```python
from build123d import *

# Parameters (mm, degrees)
SKETCH2_R           = 3.175
BOSS_EXTRUDE2_DEPTH = 25.4
SKETCH3_R           = 4.7625
CUT_EXTRUDE1_DEPTH  = 14.2875


with BuildPart() as part:
    # Sketch2 → Boss-Extrude2 (new body)
    with BuildSketch(Plane(origin=(0, 0, 0), x_dir=(1, 0, 0), z_dir=(0, 1, 0))):
        with BuildLine():
            Line((-15.875, 12.7), (-15.875, -12.7))
            Line((-15.875, -12.7), (15.875, -12.7))
            ThreePointArc((15.875, -12.7), (3.175, 0), (15.875, 12.7))
            Line((15.875, 12.7), (-15.875, 12.7))
        make_face()
        with Locations((-6.35, 0)):
            Circle(SKETCH2_R, mode=Mode.SUBTRACT)
    extrude(amount=BOSS_EXTRUDE2_DEPTH)

    # Sketch3 → Cut-Extrude1 (cut)
    with BuildSketch(Plane.ZY.offset(15.875)):
        with Locations((0, 12.7)):
            Circle(SKETCH3_R)
    extrude(amount=-CUT_EXTRUDE1_DEPTH, mode=Mode.SUBTRACT)


solid = part.part
```
Geometry check sheet. Reference: the model listing, model coordinates, mm. A direction names the side the tool comes from. Round coordinates to 2 decimals unless told otherwise and drop trailing zeros. Loops run counter-clockwise (first coordinate to the right, second up) from the corner with the lowest first, then second, coordinate; pieces in that order, holes last. Notation, with made-up numbers: M 82,46.25 L 104,46.25 A4 ccw 104,51.25 Z; hole C -25.75,49 d8. An arc over 180 degrees is marked long. Return JSON: item names as keys, results as strings. Group by question number.
(1) Mould release check, pull along Z, two halves, no side actions. Record for faces 1 (the face through (0, 13, -12.7)), 2 (the face through (-3.32, 4.51, -0.95)), 3 (the face through (-4, 0, -3)), 4 (the face through (-3.32, 20.76, -0.95)): pulls with the +Z half, pulls with the -Z half, needs draft (parallel to the pull), parting line crosses it, or undercut.
(2) Section check B-B, the plane x = -6.35. Enter the section's corners in (y, z) (1 decimal), and give its area (3 significant figures).
(3) Set-up check for faces 5 (the face through (3.18, 12.52, 0.28)), 6 (the face through (-1.588, 13, 0)): record each of +Z, -Z, +X, -X, +Y, -Y from which the full face is reachable in a straight line by a thin tool's end or side.
(4) Section check C-C, the plane y = 5. Enter the section's corners in (x, z) (3 decimals), and give its area (3 significant figures).
(5) Go/stop test with a flat-tipped pin: pin 1 (8.5 mm diameter, centred on y = 12.7, z = 0, fed in from +X). Record where the tip stops, or that it passes through.
(6) Section check D-D, the plane x = -13. Enter the section's corners in (y, z) (1 decimal).
(7) Section check A-A, the plane z = 0. Enter the section's corners in (x, y) (1 decimal), and give its area (3 significant figures).
(8) Scan lines: line 1 along X through (y, z) = (4.5, 0) (3 decimals); line 2 along Z through (x, y) = (-6.35, 3.5) (3 decimals); line 3 along Y through (x, z) = (-10, 0). Record each from-to range of solid material in increasing order. Write a range as [from, to].
Data:
{
 "1": {"face 1": "pulls with the -Z half", "face 2": "undercut", "face 3": "needs draft", "face 4": "undercut"},
 "2": {"outline": "M 0,-12.7 L 25.4,-12.7 L 25.4,-3.2 L 16.2,-3.2 A4.8 cw 9.2,-3.2 L 0,-3.2 Z; M 0,3.2 L 9.2,3.2 A4.8 cw 16.2,3.2 L 25.4,3.2 L 25.4,12.7 L 0,12.7 Z", "area": "468 mm²"},
 "3": {"face 5": "+X, +Y, -Y", "face 6": "-X"},
 "4": {"outline": "M -15.875,-12.7 L 15.875,-12.7 A12.7 cw 15.875,12.7 L -15.875,12.7 Z; hole C -6.35,0 d6.35", "area": "521 mm²"},
 "5": {"pin 1": "x = 3.91"},
 "6": {"outline": "M 0,-12.7 L 25.4,-12.7 L 25.4,12.7 L 0,12.7 Z; hole C 12.7,0 d9.5"},
 "7": {"outline": "M -15.9,0 L -9.5,0 L -9.5,7.9 L -15.9,7.9 Z; M -15.9,17.5 L -9.5,17.5 L -9.5,25.4 L -15.9,25.4 Z; M -3.2,0 L 3.2,0 L 3.2,25.4 L -3.2,25.4 L -3.2,17.5 L -1.6,17.5 L -1.6,7.9 L -3.2,7.9 Z", "area": "247 mm²"},
 "8": {"line 1": "[-15.875, -9.525], [-3.175, 3.175]", "line 2": "[-12.7, -3.175], [3.175, 12.7]", "line 3": "[0, 7.94], [17.46, 25.4]"}
}
